Verification items for the finished model (mm, model axes). Round coordinates to 2 decimals unless told otherwise and drop trailing zeros. Write each loop counter-clockwise with the first axis right and the second up, starting at its lowest first coordinate (ties: lowest second). Pieces come first, ordered by that corner, then holes. Notation, with made-up numbers: (-5, -38.5) -> (42, -38.5) arc R6 ccw to (42, -30.5) -> close; hole circle Ø6 at (19.25, -34.5). An arc over 180 degrees is marked (long way). Use CSV: the item, a comma, the result in double quotes.
```python
from build123d import *

# Parameters (mm, degrees)
F0_R     = 29.567188
F1_DEPTH = 31.353125
F2_R     = 0.508
F3_R     = 29.567188
F4_DEPTH = 19.446875
F5_R     = 0.508


with BuildPart() as f1:
    # F0 (on Top) → F1 (new body)
    with BuildSketch(Plane.XY):
        Circle(F0_R)
    extrude(amount=F1_DEPTH)

    # F2
    f2_edges = [f1.edges().sort_by_distance(p)[0] for p in [
        (-29.567188, 0, 0),
        (-29.567188, 0, 31.353125),
    ]]
    fillet(f2_edges, radius=F2_R)

    # F3 (on face) → F4 (join)
    with BuildSketch(Plane.XY.offset(31.353125)):
        Circle(F3_R)
    extrude(amount=F4_DEPTH)

    # F5
    f5_edges = [f1.edges().sort_by_distance(p)[0] for p in [
        (-29.567188, 0, 50.8),
    ]]
    fillet(f5_edges, radius=F5_R)


solid = f1.part
```
Q1. Go/stop test with flat-tipped pins: P1, Ø2, axis at x = 8, z = 7, coming from the +Y side; P2, Ø2, axis at y = 11, z = 8, coming from the -X side; P3, Ø5, axis at y = -13, z = 21, coming from the -X side. Record where each tip stops, or that it passes through.
Filled in:
P1,"y = 28.73"
P2,"x = -27.82"
P3,"x = -27.64"
Q2. Material ranges on L1, parallel to X at y = 0.5, z = 35.5; L2, parallel to Y at x = 0, z = 36; L3, parallel to Y at x = -10.5, z = 40.5, recorded low to high.
Filled in:
L1,"-29.56 to 29.56"
L2,"-29.57 to 29.57"
L3,"-27.64 to 27.64"
Q3. Section check A-A (z = 11). Record the cut outline in (x, y).
Filled in:
outline,"circle Ø59.13 at (0, 0)"
